Geometry: final body of the model. Coordinates: model frame, mm. Face numbers are marked on the shaded views. A direction names the side the tool comes from. Give positions to 0.01 mm unless a question says otherwise; leave off trailing zeros. Loops run counter-clockwise (first coordinate to the right, second up) from the corner with the lowest first, then second, coordinate; pieces in that order, holes last.
1. Section A-A, the plane y = 1.5. Output: boundary loops of the cut face in (x, z), then the cut area to 3 significant figures.
2. Material intervals for line 1 along X through (y, z) = (7, -13.5) (3 decimals); line 2 along X through (y, z) = (7.65, 13.5) (3 decimals); line 3 along X through (y, z) = (8.75, -5.5), sorted ascending.
3. Access query for the marked faces 1, 2 and 3. Directions: +Z, -Z, +X, -X, +Y, -Y. A direction counts if a zero-diameter tool reaches every point of the face in a straight line with its end or side. Return the directions, or none.
4. Section C-C, the plane x = 1. Output: boundary loops of the cut face in (y, z), then the cut area to 3 significant figures.
5. Section D-D, the plane z = -13.5. Output: boundary loops of the cut face in (x, y) (3 decimals), then the cut area to 3 significant figures.
6. First-contact query: P1, Ø14.5, axis at x = 2, z = 2, coming from the +Y side; P2, Ø2.5, axis at x = 10, z = 13.5, coming from the +Y side. Flat tips, straight axial feed; report the tip coordinate or a pass-through.
7. Section B-B, the plane z = -4. Output: boundary loops of the cut face in (x, y).
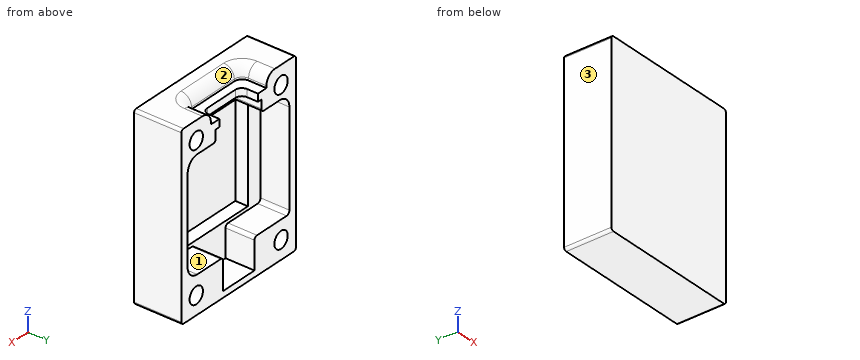
from build123d import *

# Parameters (mm, degrees)
SKETCH_1_W          = 27
SKETCH_1_H          = 34
EXTRUDE_1_DEPTH     = 9
CUT_EXTRUDE_1_DEPTH = 5.5
SKETCH_5_W          = 18
SKETCH_5_H          = 20
CUT_EXTRUDE_2_DEPTH = 2.4
SKETCH_7_W          = 9.1
SKETCH_7_H          = 3.3
CUT_EXTRUDE_3_DEPTH = 3.820001
CUT_EXTRUDE_4_DEPTH = 2.4
SKETCH_9_R          = 1.575
CUT_EXTRUDE_5_DEPTH = 3.1
FILLET_1_R          = 0.5
FILLET_2_R          = 1.5
FILLET_3_R          = 1.25
FILLET_4_R          = 2


with BuildPart() as part:
    # 草图1 → 凸台-拉伸1 (new body)
    with BuildSketch(Plane(origin=(0, 0, 0), x_dir=(1, 0, 0), z_dir=(0, 1, 0))):
        Rectangle(SKETCH_1_W, SKETCH_1_H)
    extrude(amount=EXTRUDE_1_DEPTH)

    # 草图3 → 切除-拉伸1 (cut)
    with BuildSketch(Plane(origin=(0, 9, 0), x_dir=(1, 0, 0), z_dir=(0, 1, 0))):
        with BuildLine():
            Line((-3.725034324, 15.819299777), (3.648970913, 15.819299777))
            Line((3.648970913, 15.819299777), (3.64896994, 10.554745119))
            ThreePointArc((3.64896994, 10.554745119), (3.822350515, 10.139234755), (4.241249073, 9.974209696))
            Line((4.241249073, 9.974209696), (9.783400257, 9.974209696))
            ThreePointArc((9.783400257, 9.974209696), (11.370154466, 9.295205446), (12.02766691, 7.699425674))
            Line((12.02766691, 7.699425674), (12.02766691, -8.683574325))
            ThreePointArc((12.02766691, -8.683574325), (11.356679802, -10.306708388), (9.731381036, -10.972434915))
            Line((9.731381036, -10.972434915), (5.988537145, -10.972434915))
            ThreePointArc((5.988537145, -10.972434915), (5.590573679, -11.145336005), (5.425084588, -11.546438321))
            Line((5.425084588, -11.546438321), (5.425084588, -13.179999201))
            Line((5.425084588, -13.179999201), (-5.361915412, -13.179999201))
            Line((-5.361915412, -13.179999201), (-5.361915412, -11.557540546))
            ThreePointArc((-5.361915412, -11.557540546), (-5.529636352, -11.146058241), (-5.93984312, -10.975241356))
            Line((-5.93984312, -10.975241356), (-9.683907212, -10.975243852))
            ThreePointArc((-9.683907212, -10.975243852), (-11.295675804, -10.308730473), (-11.96592401, -8.698511128))
            Line((-11.96592401, -8.698511128), (-11.965923922, 9.282882934))
            ThreePointArc((-11.965923922, 9.282882934), (-11.776218419, 9.756882394), (-11.311023769, 9.967257479))
            Line((-11.311023769, 9.967257479), (-4.318854243, 9.967257479))
            ThreePointArc((-4.318854243, 9.967257479), (-3.899962458, 10.130736448), (-3.725034039, 10.544977621))
            Line((-3.725034039, 10.544977621), (-3.725034324, 15.819299777))
        make_face()
    extrude(amount=-CUT_EXTRUDE_1_DEPTH, mode=Mode.SUBTRACT)

    # 草图5 → 切除-拉伸2 (cut)
    with BuildSketch(Plane(origin=(0, 3.5, 0), x_dir=(1, 0, 0), z_dir=(0, 1, 0))):
        with Locations((0, -0.680700223)):
            Rectangle(SKETCH_5_W, SKETCH_5_H)
    extrude(amount=-CUT_EXTRUDE_2_DEPTH, mode=Mode.SUBTRACT)

    # 草图7 → 切除-拉伸3 (cut)
    with BuildSketch(Plane.XY.offset(17)):
        with Locations((0, 7.35)):
            Rectangle(SKETCH_7_W, SKETCH_7_H)
    extrude(amount=-CUT_EXTRUDE_3_DEPTH, mode=Mode.SUBTRACT)

    # 草图8 → 切除-拉伸4 (cut)
    with BuildSketch(Plane.XY.offset(17)):
        Polygon((6.55, 4.1), (-6.55, 4.1), (-6.55, 9), (-4.55, 9), (4.55, 9), (6.55, 9), align=None)
    extrude(amount=-CUT_EXTRUDE_4_DEPTH, mode=Mode.SUBTRACT)

    # 草图9 → 切除-拉伸5 (cut)
    with BuildSketch(Plane(origin=(0, 9, 0), x_dir=(1, 0, 0), z_dir=(0, 1, 0))):
        with Locations((-10, 13.5)):
            Circle(SKETCH_9_R)
        with Locations((10, 13.5)):
            Circle(SKETCH_9_R)
        with Locations((10, -13.5)):
            Circle(SKETCH_9_R)
        with Locations((-10, -13.5)):
            Circle(SKETCH_9_R)
    extrude(amount=-CUT_EXTRUDE_5_DEPTH, mode=Mode.SUBTRACT)

    # 圆角1
    fillet_1_edges = [part.edges().sort_by_distance(p)[0] for p in [
        (13.5, 4.5, 17),
        (-13.5, 4.5, 17),
        (-13.5, 4.5, -17),
        (13.5, 4.5, -17),
    ]]
    fillet(fillet_1_edges, radius=FILLET_1_R)

    # 圆角2
    fillet_2_edges = [part.edges().sort_by_distance(p)[0] for p in [
        (6.55, 4.1, 15.8),
        (-6.55, 4.1, 15.8),
    ]]
    fillet(fillet_2_edges, radius=FILLET_2_R)

    # 圆角3
    fillet_3_edges = [part.edges().sort_by_distance(p)[0] for p in [
        (4.55, 5.7, 13.8899995),
        (-4.55, 5.7, 13.8899995),
    ]]
    fillet(fillet_3_edges, radius=FILLET_3_R)

    # 圆角4
    fillet_4_edges = [part.edges().sort_by_distance(p)[0] for p in [
        (-6.55, 7.3, 17),
        (6.55, 7.3, 17),
        (0, 4.1, 17),
        (6.110660172, 4.539339828, 17),
        (-6.110660172, 4.539339828, 17),
    ]]
    fillet(fillet_4_edges, radius=FILLET_4_R)


solid = part.part
Answers below:
1. outline: (-13.5, -16.5) arc R0.5 ccw to (-13, -17) - (13, -17) arc R0.5 ccw to (13.5, -16.5) - (13.5, 16.5) arc R0.5 ccw to (13, 17) - (-13, 17) arc R0.5 ccw to (-13.5, 16.5) - close; hole (-9, -9.32) - (9, -9.32) - (9, 10.68) - (-9, 10.68) - close
1. area: 558 mm2
2. line 1: x = -13.5 to -11.575, -8.425 to -3.725, 3.649 to 8.425, 11.575 to 13.5
2. line 2: x = -13.5 to -11.575, -8.425 to -4.55, 4.55 to 8.425, 11.575 to 13.5
2. line 3: x = -13.5 to -11.97, 12.03 to 13.5
3. face 1: +Y
3. face 2: +Z, +Y
3. face 3: +Z, -Z, -X, +Y, -Y
4. outline: (0, -17) - (9, -17) - (9, -15.82) - (3.5, -15.82) - (3.5, -9.32) - (1.1, -9.32) - (1.1, 10.68) - (3.5, 10.68) - (3.5, 13.18) - (5.7, 13.18) - (5.7, 14.6) - (4.1, 14.6) - (4.1, 15) arc R2 ccw to (2.1, 17) - (0, 17) - close
4. area: 81.2 mm2
5. outline: (-13.5, 0) - (13.5, 0) - (13.5, 9) - (11.575, 9) - (11.575, 5.9) - (8.425, 5.9) - (8.425, 9) - (3.649, 9) - (3.649, 3.5) - (-3.725, 3.5) - (-3.725, 9) - (-8.425, 9) - (-8.425, 5.9) - (-11.575, 5.9) - (-11.575, 9) - (-13.5, 9) - close
5. area: 183 mm2
6. P1: stops at y = 3.5
6. P2: stops at y = 5.9
7. outline: (-13.5, 0) - (13.5, 0) - (13.5, 9) - (12.03, 9) - (12.03, 3.5) - (9, 3.5) - (9, 1.1) - (-9, 1.1) - (-9, 3.5) - (-11.97, 3.5) - (-11.97, 9) - (-13.5, 9) - close
